Geometry check sheet. Reference: the model listing, model coordinates, mm. A direction names the side the tool comes from. Give positions to 0.01 mm unless a question says otherwise; leave off trailing zeros. Order: outer loops, then holes, each group sorted by start corner. A loop starts at its lowest first (then second) coordinate and runs counter-clockwise, first axis right, second up.
```python
from build123d import *

# Parameters (mm, degrees)
F0_W      = 36.576
F0_H      = 30.226
F0_W_2    = 25.908
F0_H_2    = 19.558
F1_DEPTH  = 15.875
F2_W      = 12.446
F2_H      = 6.096
F3_DEPTH  = 31.75
F4_W      = 88.9
F4_H      = 12.7
F5_DEPTH  = 19.05
F7_DEPTH  = 6.35
F9_R      = 3
F10_DEPTH = 30.227


with BuildPart() as f1:
    # F0 (on Top) → F1 (new body, symmetric)
    with BuildSketch(Plane.XY):
        Rectangle(F0_W, F0_H)
        Rectangle(F0_W_2, F0_H_2, mode=Mode.SUBTRACT)
    extrude(amount=F1_DEPTH, both=True)

    # F2 (on face) → F3 (join)
    with BuildSketch(Plane.XY.offset(15.875)):
        with Locations((0, 6.731)):
            Rectangle(F2_W, F2_H)
    extrude(amount=-F3_DEPTH)

    # F4 (on face) → F5 (join)
    with BuildSketch(Plane(origin=(0, 0, -15.875), x_dir=(1, 0, 0), z_dir=(0, 0, -1))):
        with Locations((62.738, 8.763)):
            Rectangle(F4_W, F4_H)
    extrude(amount=-F5_DEPTH)

    # F6 (on face) → F7 (join)
    with BuildSketch(Plane.XZ.offset(15.113)):
        Polygon((43.688, 3.175), (18.288, 15.875), (18.288, 3.175), align=None)
    extrude(amount=-F7_DEPTH)

    # F9 (on face) → F10 (cut, through all)
    with BuildSketch(Plane.XZ.offset(15.113)):
        Circle(F9_R)
    extrude(amount=-F10_DEPTH, mode=Mode.SUBTRACT)


solid = f1.part
```
Q1. Cross-section at D-D, the plane z = 0. Record the boundary of the cut face in (x, y).
Q2. Cross-section at B-B, the plane x = 0. Record the boundary of the cut face in (y, z) (3 decimals).
Q3. Thickness scan on L1, parallel to X at y = 6, z = 9.5; L2, parallel to Y at x = -7, z = 2; L3, parallel to Y at x = -2, z = 8.5. Record the ranges inside material, lowest first.
Q4. Gauge pin test, flat ends, axial feed: P1, Ø8, axis at x = 5.5, y = -3, coming from the -Z side; P2, Ø2, axis at y = 6, z = -0.5, coming from the +X side; P3, Ø9.5, axis at x = 44.5, z = -3, coming from the +Y side; P4, Ø4, axis at x = 28.5, z = 9.5, coming from the +Y side. Record the tip position at first contact, or that the pin passes through.
Q5. Release check for a two-part mould opening along Y. For faces 4 (the face through (-6.223, 7, 0)), 5 (the face through (10, 9.779, 0)), 6 (the face through (62, -2.413, -6)), 7 (the face through (18.288, 3, 0)) record: pulls with the +Y half, pulls with the -Y half, needs draft (parallel to the pull), parting line crosses it, or undercut.
Q6. Access from +Z, -Z, +X, -X, +Y, -Y to the whole of each face (thin tool, end or side, straight path). Record for faces 1 (the face through (12.954, 0, 0)), 2 (the face through (72, -9, 3.175)), 3 (the face through (107.188, -9, -6)).
Q7. Cross-section at A-A, the plane y = 8.5. Record the boundary of the cut face in (x, z) (3 decimals).
Q8. Cross-section at C-C, the plane y = 2. Record the boundary of the cut face in (x, z) (3 decimals).
Answers follow:
1. outline: (-18.29, -15.11) - (-3, -15.11) - (-3, -9.78) - (-12.95, -9.78) - (-12.95, 9.78) - (-6.22, 9.78) - (-6.22, 3.68) - (-3, 3.68) - (-3, 15.11) - (-18.29, 15.11) - close; (3, -15.11) - (107.19, -15.11) - (107.19, -2.41) - (18.29, -2.41) - (18.29, 15.11) - (3, 15.11) - (3, 3.68) - (6.22, 3.68) - (6.22, 9.78) - (12.95, 9.78) - (12.95, -9.78) - (3, -9.78) - close
2. outline: (-15.113, -15.875) - (-9.779, -15.875) - (-9.779, -3) - (-15.113, -3) - close; (-15.113, 3) - (-9.779, 3) - (-9.779, 15.875) - (-15.113, 15.875) - close; (3.683, -15.875) - (15.113, -15.875) - (15.113, -3) - (3.683, -3) - close; (3.683, 3) - (15.113, 3) - (15.113, 15.875) - (3.683, 15.875) - close
3. L1: x = -18.29 to -12.95, -6.22 to 6.22, 12.95 to 18.29
3. L2: y = -15.11 to -9.78, 9.78 to 15.11
3. L3: y = -15.11 to -9.78, 3.68 to 15.11
4. P1: passes through
4. P2: stops at x = 18.29
4. P3: stops at y = -2.41
4. P4: stops at y = -8.76
5. face 4: undercut
5. face 5: undercut
5. face 6: pulls with the +Y half
5. face 7: needs draft
6. face 1: +Z, -Z
6. face 2: +Z, +X, +Y
6. face 3: +Z, -Z, +X, +Y, -Y
7. outline: (-18.288, -15.875) - (-12.954, -15.875) - (-12.954, 15.875) - (-18.288, 15.875) - close; (-6.223, -15.875) - (6.223, -15.875) - (6.223, 15.875) - (-6.223, 15.875) - close; (12.954, -15.875) - (18.288, -15.875) - (18.288, 15.875) - (12.954, 15.875) - close; hole circle Ø6 at (0, 0)
8. outline: (-18.288, -15.875) - (-12.954, -15.875) - (-12.954, 15.875) - (-18.288, 15.875) - close; (12.954, -15.875) - (18.288, -15.875) - (18.288, 15.875) - (12.954, 15.875) - close
